```python
from build123d import *

# Parameters (mm, degrees)
PAD_DEPTH     = 10
SKETCH001_R   = 7.5
HOLE_DEPTH    = 10.001
SKETCH003_R   = 10.5
HOLE002_DEPTH = 5
PAD001_DEPTH  = 2
SKETCH005_R   = 2.2
HOLE003_DEPTH = 12.001


with BuildPart() as part:
    # Sketch → Pad (new body)
    with BuildSketch(Plane.YZ):
        with BuildLine():
            ThreePointArc((-17.5, 0), (1.8e-05, -17.5), (17.5, 3.6e-05))
            Line((17.5, 3.6e-05), (17.5, 67.5))
            Line((-17.5, 67.5), (17.5, 67.5))
            Line((-17.5, 0), (-17.5, 67.5))
        make_face()
    extrude(amount=-PAD_DEPTH)

    # Sketch001 (on Face5 of Pad) → Hole (cut, through all)
    with BuildSketch(Plane.YZ):
        Circle(SKETCH001_R)
    extrude(amount=-HOLE_DEPTH, mode=Mode.SUBTRACT)

    # Sketch003 → Hole002 (cut)
    with BuildSketch(Plane(origin=(-10, 0, 0), x_dir=(0, 1, 0), z_dir=(-1, 0, 0))):
        Circle(SKETCH003_R)
    extrude(amount=-HOLE002_DEPTH, mode=Mode.SUBTRACT)

    # Sketch004 (on Face6 of Pad) → Pad001 (join)
    with BuildSketch(Plane(origin=(-10, 0, 0), x_dir=(0, 1, 0), z_dir=(-1, 0, 0))):
        with BuildLine():
            Line((-17.5, -35.968736), (-17.5, -67.5))
            Line((-17.5, -67.5), (17.5, -67.5))
            Line((17.5, -67.5), (17.5, -35.968736))
            ThreePointArc((13.919411, -37.5), (15.728351, -36.777968), (17.5, -35.968736))
            Line((-13.919411, -37.5), (13.919411, -37.5))
            ThreePointArc((-17.5, -35.968736), (-15.728351, -36.777968), (-13.919411, -37.5))
        make_face()
    extrude(amount=PAD001_DEPTH)

    # Sketch005 (on Face15 of Pad001) → Hole003 (cut, through all)
    with BuildSketch(Plane(origin=(-12, 0, 0), x_dir=(0, 1, 0), z_dir=(-1, 0, 0))):
        with Locations((-10.5, -44.5)):
            Circle(SKETCH005_R)
        with Locations((-10.5, -60.5)):
            Circle(SKETCH005_R)
        with Locations((10.5, -44.5)):
            Circle(SKETCH005_R)
        with Locations((10.5, -60.5)):
            Circle(SKETCH005_R)
    extrude(amount=-HOLE003_DEPTH, mode=Mode.SUBTRACT)


solid = part.part
```
Source: CAD feature listing. Evaluate the final solid. Frame: model axes, mm. A direction names the side the tool comes from. Coordinates: 2 decimals unless noted, no trailing zeros. Order: outer loops, then holes, each group sorted by start corner. A loop starts at its lowest first (then second) coordinate and runs counter-clockwise, first axis right, second up. Notation, with made-up numbers: M 30.5,-35.5 L 61.5,-35.5 A25 ccw 61.5,-18.5 Z; hole C -3.5,77 d11. An arc over 180 degrees is marked long. Write each question's results on one line, items separated by ' | '. Start each with the question number.
1) Section query C-C (x = -1.75). Return the cut outline in (y, z), plus the area to 3 significant figures.
2) Access query for faces 1 (the face through (-6.084, -10.977, 62.648)), 2 (the face through (-5, 5, 7)), 3 (the face through (-10.99, -15.75, 36.77)). Directions: +Z, -Z, +X, -X, +Y, -Y. A direction counts if a zero-diameter tool reaches every point of the face in a straight line with its end or side. Return the directions, or none.
3) Draft query along Z for faces 4 (the face through (-10, 0, 16)), 5 (the face through (-10.99, 15.7, 36.79)), 6 (the face through (-7.5, 10, -3.2)), 7 (the face through (-2.465, -7.493, 0.33)). Return one class per face: released by +Z, released by -Z, zero draft, split by the parting line, or undercut.
4) Section query B-B (z = 44.5). Return the cut outline in (x, y), plus the area to 3 significant figures.
5) Section query D-D (z = -2). Return the cut outline in (x, y).
6) Line query: line 1 (Y direction, x = -3, z = 60.5); line 2 (Z direction, x = -2.8, y = 0); line 3 (Y direction, x = -6.25, z = 43.5). Output: solid intervals per line, ascending. Write a range as from..to.
7) Section query A-A (y = 0). Return the cut outline in (x, z).
8) Contact query for flat-ended pins moving along their axis: pin 1 Ø1.6 at (x, y) = (-11, 6) entering from -Z; pin 2 Ø17 at (y, z) = (-3, 1) entering from -X; pin 3 Ø5.5 at (y, z) = (10.5, 60.5) entering from -X. Output: stop coordinate, or through.
Answers:
1) outline: M -17.5,0 A17.5 ccw 17.5,0 L 17.5,67.5 L -17.5,67.5 Z; hole C -10.5,44.5 d4.4; hole C -10.5,60.5 d4.4; hole C 0,0 d15; hole C 10.5,44.5 d4.4; hole C 10.5,60.5 d4.4 | area: 2,610 mm^2
2) face 1: +X, -X | face 2: -X | face 3: -Z, -X
3) face 4: zero draft | face 5: released by -Z | face 6: undercut | face 7: undercut
4) outline: M -12,-17.5 L 0,-17.5 L 0,-12.7 L -12,-12.7 Z; M -12,-8.3 L 0,-8.3 L 0,8.3 L -12,8.3 Z; M -12,12.7 L 0,12.7 L 0,17.5 L -12,17.5 Z | area: 314 mm^2
5) outline: M -10,-17.39 L 0,-17.39 L 0,-7.23 L -5,-7.23 L -5,-10.31 L -10,-10.31 Z; M -10,10.31 L -5,10.31 L -5,7.23 L 0,7.23 L 0,17.39 L -10,17.39 Z
6) line 1: y = -17.5..-12.7, -8.3..8.3, 12.7..17.5 | line 2: z = -17.5..-7.5, 7.5..67.5 | line 3: y = -17.5..-12.46, -8.54..8.54, 12.46..17.5
7) outline: M -12,37.5 L -10,37.5 L -10,10.5 L -5,10.5 L -5,7.5 L 0,7.5 L 0,67.5 L -12,67.5 Z; M -10,-17.5 L 0,-17.5 L 0,-7.5 L -5,-7.5 L -5,-10.5 L -10,-10.5 Z
8) pin 1: stops at z = 37.5 | pin 2: stops at x = -10 | pin 3: stops at x = -12
